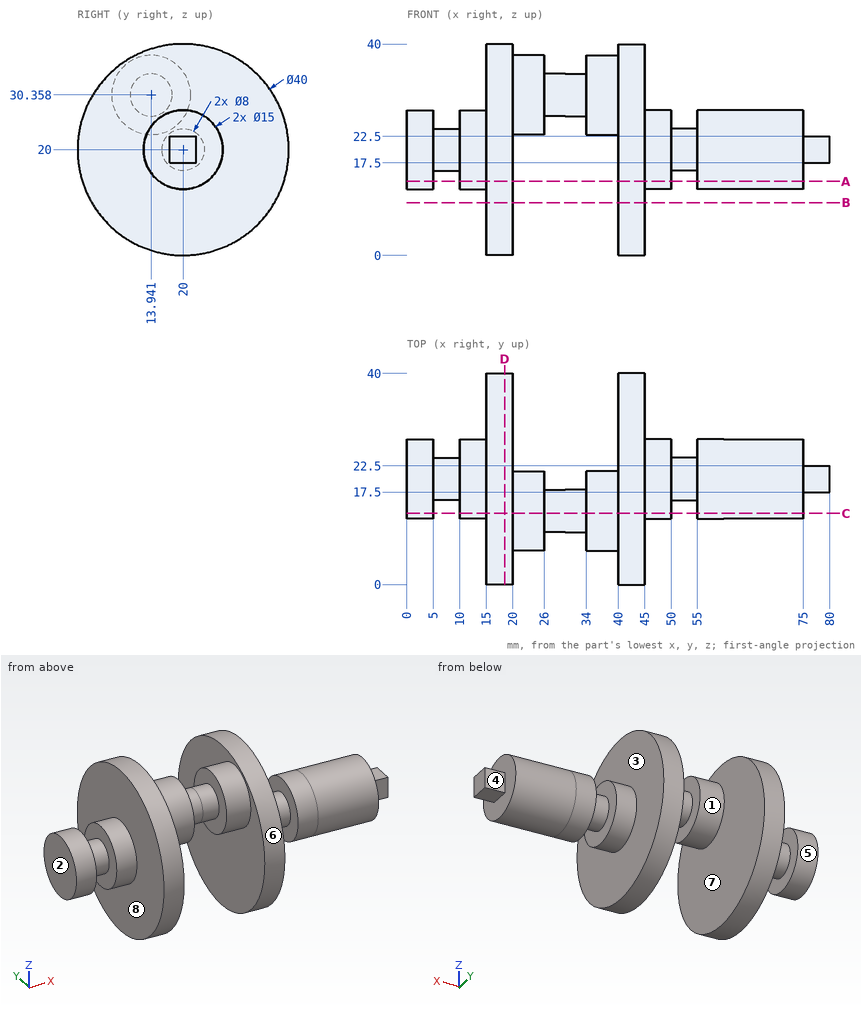
Input: dimensioned drawing with shaded views. Units: mm. Origin: part minimum x, y, z. A direction names the side the tool comes from. Give positions to 0.01 mm unless a question says otherwise; leave off trailing zeros. Loops run counter-clockwise (first coordinate to the right, second up) from the corner with the lowest first, then second, coordinate; pieces in that order, holes last. Notation, with made-up numbers: (50.25, 75) - (106.25, 75) arc R21 cw to (106.25, 88) - close; hole circle Ø2 at (23, 30). An arc over 180 degrees is marked (long way). Answer as CSV lines item,"result". Start each with the question number.
(1) Section query B-B (z = 10). Output: boundary loops of the cut face in (x, y).
(2) Reachability of the marked faces 1, 2, 3, 4 and 5 from +Z, -Z, +X, -X, +Y, -Y: full face, straight path, thin tool, end or side. Return the list, or none.
(3) Section query A-A (z = 14). Output: boundary loops of the cut face in (x, y).
(4) Section query C-C (y = 13.5). Give the number of separate pieces and of enclosed holes in the cut face.
(5) Ray query, line 1 along X through (y, z) = (21, 10); line 2 along X through (y, z) = (22, 20.5); line 3 along X through (y, z) = (13, 29.5). Return the intervals inside material, ascending. Write a range as [from, to].
(6) Pin query (flat end, axial travel): P1, Ø3, axis at x = 29, z = 36, coming from the -Y side; P2, Ø12, axis at y = 12.5, z = 28, coming from the +X side; P3, Ø12, axis at x = 65, z = 21.5, coming from the +Y side; P4, Ø2.5, axis at x = 77.5, z = 21, coming from the +Y side. Return the tip coordinate at first contact, or that it passes through.
(7) Mould query, pull axis X, two halves, no side actions, for the marked faces 6, 7 and 8. Classes: +X half, -X half, draft (parallel to the pull), parting line (faces both ways), or undercut.
(8) Section query D-D (x = 18.5). Output: boundary loops of the cut face in (y, z), and give its area (3 significant figures).
Worked answers:
1,outline,"(15, 2.68) - (20, 2.68) - (20, 37.32) - (15, 37.32) - close; (40, 2.68) - (45, 2.68) - (45, 37.32) - (40, 37.32) - close"
2,face 1,"none"
2,face 2,"+Z, -Z, -X, +Y, -Y"
2,face 3,"+X"
2,face 4,"+Z, -Z, +X, +Y"
2,face 5,"-X"
3,outline,"(0, 15.5) - (5, 15.5) - (5, 24.5) - (0, 24.5) - close; (10, 15.5) - (15, 15.5) - (15, 0.92) - (20, 0.92) - (20, 39.08) - (15, 39.08) - (15, 24.5) - (10, 24.5) - close; (40, 0.92) - (45, 0.92) - (45, 15.5) - (50, 15.5) - (50, 24.5) - (45, 24.5) - (45, 39.08) - (40, 39.08) - close; (55, 15.5) - (75, 15.5) - (75, 24.5) - (55, 24.5) - close"
4,separate pieces,"3"
4,enclosed holes,"0"
5,line 1,"x = [15, 20], [40, 45]"
5,line 2,"x = [0, 20], [40, 80]"
5,line 3,"x = [15, 45]"
6,P1,"passes through"
6,P2,"stops at x = 75"
6,P3,"stops at y = 27.5"
6,P4,"stops at y = 22.5"
7,face 6,"draft"
7,face 7,"undercut"
7,face 8,"-X half"
8,outline,"circle Ø40 at (20, 20)"
8,area,"1,260 mm^2"
